The listing builds one solid part. Answer for the finished solid, in the listing's coordinates (mm). A direction names the side the tool comes from. Round coordinates to 2 decimals unless told otherwise and drop trailing zeros. Write each loop counter-clockwise with the first axis right and the second up, starting at its lowest first coordinate (ties: lowest second). Pieces come first, ordered by that corner, then holes.
(1) Find the intervals of material crossed by probe 1 along X at (y, z) = (-11.5, 9.75); probe 2 along Y at (x, z) = (4, 2.25); probe 3 along Y at (x, z) = (15.65, 5), in increasing order.
(2) Each of these flat-tipped pins is pushed along its axis until it touches: pin 1 Ø5 at (y, z) = (-10.5, 5) entering from -X; pin 2 Ø3 at (y, z) = (-47, 7.5) entering from -X; pin 3 Ø0.6 at (y, z) = (-84.5, 0.5) entering from -X. Where does it stop, or does it pass through?
(3) A cutting plane is placed at C-C, the plane z = 5. Give the number of separate pieces and of enclosed holes in the cut face, and give its area (3 significant figures).
(4) A cutting plane is placed at B-B, the plane y = 10. Give the vertices of the cut face in (x, z), and give its area (3 significant figures).
(5) A cutting plane is placed at A-A, the plane y = -10.5. Give the vertices of the cut face in (x, z).
(6) For faces 4 (the face through (15.33, 39.996, 2.708)), 5 (the face through (9, -3, 5)), 6 (the face through (6.844, -85.028, 6.508)), determine the directions among +Z, -Z, +X, -X, +Y, -Y from which every point of the face is accessible in a straight line to the end or side of a thin tool.
(7) The mould has two halves that part along Y. Classify faces 1 (the face through (-0.15, 39.99, 5.07)), 2 (the face through (-0.15, 0.01, 5.07)), 3 (the face through (13.6, -2.4, 10)): +Y half, -Y half, draft (parallel to the pull), parting line (faces both ways), or undercut.
from build123d import *

# Parameters (mm, degrees)
BOSS_EXTRUDE2_DEPTH      = 10
CUT_EXTRUDE2_DEPTH       = 90.877694674
CUT_EXTRUDE2_DEPTH_BACK  = 90.877694674
SKETCH5_W                = 11
SKETCH5_H                = 67.407766248
CUT_EXTRUDE3_DEPTH       = 87.446515257
CUT_EXTRUDE3_DEPTH_BACK  = 87.446515257
SKETCH16_R               = 1.85
FILLET16_R               = 15
CUT_EXTRUDE20_DEPTH      = 92.021975369
CUT_EXTRUDE20_DEPTH_BACK = 92.021975369
SKETCH45_R               = 1.85
SKETCH52_W               = 15
SKETCH52_H               = 10
BOSS_EXTRUDE25_DEPTH     = 4
FILLET17_R               = 10
FILLET18_R               = 2
SKETCH53_R               = 1.9
CUT_EXTRUDE25_DEPTH      = 10
SKETCH55_W               = 0.5
SKETCH55_H               = 4
CUT_EXTRUDE28_DEPTH      = 10
CUT_EXTRUDE32_DEPTH      = 91.055538419
CUT_EXTRUDE32_DEPTH_BACK = 91.055538419
SKETCH60_R               = 2
FILLET19_R               = 10
SKETCH61_R               = 1.85
CUT_EXTRUDE33_DEPTH      = 10


with BuildPart() as part:
    # Sketch2 → Boss-Extrude2 (new body)
    with BuildSketch(Plane.XY):
        Polygon((18, -3), (33, -3), (33, 43), (-3, 43), (-3, -3), (11, -3), (11, -83), (18, -83), align=None)
        Polygon((15, 0), (30, 0), (30, 40), (0, 40), (0, 0), (14, 0), (14, -80), (15, -80), align=None, mode=Mode.SUBTRACT)
    extrude(amount=BOSS_EXTRUDE2_DEPTH)

    # Sketch5 → Cut-Extrude2 (cut, two sides: drawn at the far end of the back side and taken through both)
    with BuildSketch(Plane.XY.offset(10).offset(-CUT_EXTRUDE2_DEPTH_BACK)):
        with Locations((9.5, -51.703883124)):
            Rectangle(SKETCH5_W, SKETCH5_H)
    extrude(amount=CUT_EXTRUDE2_DEPTH + CUT_EXTRUDE2_DEPTH_BACK, mode=Mode.SUBTRACT)

    # Sketch16 → Cut-Extrude3 (cut, two sides: drawn at the far end of the back side and taken through both)
    with BuildSketch(Plane.ZY.offset(-11).offset(-CUT_EXTRUDE3_DEPTH_BACK)):
        with Locations((5, -10.5)):
            Circle(SKETCH16_R)
    extrude(amount=CUT_EXTRUDE3_DEPTH + CUT_EXTRUDE3_DEPTH_BACK, mode=Mode.SUBTRACT)

    # Fillet16
    # the kernel refuses this fillet: 15 mm, written as the material it adds along each edge
    with BuildSketch(Plane(origin=(0, 40, 0), x_dir=(0, -1, 0), z_dir=(0, 0, 1)), Plane(origin=(30, 40, 0), x_dir=(-1, 0, 0), z_dir=(0, 0, 1)), Plane(origin=(30, 0, 0), x_dir=(0, 1, 0), z_dir=(0, 0, 1))) as fillet16_piece_1:
        with BuildLine():
            CenterArc((FILLET16_R, FILLET16_R), FILLET16_R, 180, 90)
            Line((0, FILLET16_R), (-FILLET16_R * 0.02, FILLET16_R))
            Line((-FILLET16_R * 0.02, FILLET16_R), (-FILLET16_R * 0.02, -FILLET16_R * 0.02))
            Line((-FILLET16_R * 0.02, -FILLET16_R * 0.02), (FILLET16_R, -FILLET16_R * 0.02))
            Line((FILLET16_R, -FILLET16_R * 0.02), (FILLET16_R, 0))
        make_face()
    extrude(amount=10)
    with BuildSketch(Plane(origin=(0, 0, 0), x_dir=(1, 0, 0), z_dir=(0, 0, 1))) as fillet16_piece_2:
        with BuildLine():
            CenterArc((15, 14.966629547), FILLET16_R, 180, 86.177446271)
            Line((0, 14.966629547), (-0.3, 14.966629547))
            Line((-0.3, 14.966629547), (-0.3, 0))
            Line((-0.3, 0), (0, -0.3))
            ThreePointArc((0, -0.3), (7, -0.3), (13.98, -0.299332591))
            Line((13.98, -0.299332591), (14, 0))
        make_face()
    extrude(amount=10)

    # Sketch45 → Cut-Extrude20 (cut, two sides: drawn at the far end of the back side and taken through both)
    with BuildSketch(Plane.ZY.offset(3).offset(-CUT_EXTRUDE20_DEPTH_BACK)):
        with Locations((5, 20)):
            Circle(SKETCH45_R)
    extrude(amount=CUT_EXTRUDE20_DEPTH + CUT_EXTRUDE20_DEPTH_BACK, mode=Mode.SUBTRACT)

    # Sketch52 → Boss-Extrude25 (add)
    with BuildSketch(Plane.XZ.offset(83)):
        with Locations((10.5, 5)):
            Rectangle(SKETCH52_W, SKETCH52_H)
    extrude(amount=BOSS_EXTRUDE25_DEPTH)

    # Fillet17
    fillet17_edges = [part.edges().sort_by_distance(p)[0] for p in [
        (-3, -3, 5),
        (33, -3, 5),
    ]]
    fillet(fillet17_edges, radius=FILLET17_R)

    # Fillet18
    fillet18_edges = [part.edges().sort_by_distance(p)[0] for p in [
        (18, -87, 5),
    ]]
    fillet(fillet18_edges, radius=FILLET18_R)

    # Sketch53 → Cut-Extrude25 (cut)
    with BuildSketch(Plane.XZ.offset(87)):
        with Locations(Location((8, 5, 0), (0, 0, 270))):
            Circle(SKETCH53_R)
    extrude(amount=-CUT_EXTRUDE25_DEPTH, mode=Mode.SUBTRACT)

    # Sketch55 → Cut-Extrude28 (cut)
    with BuildSketch(Plane.ZY.offset(-3)):
        with Locations((0.25, -85)):
            Rectangle(SKETCH55_W, SKETCH55_H)
    extrude(amount=-CUT_EXTRUDE28_DEPTH, mode=Mode.SUBTRACT)

    # Sketch60 → Cut-Extrude32 (cut, two sides: drawn at the far end of the back side and taken through both)
    with BuildSketch(Plane(origin=(18, 0, 0), x_dir=(0, 0, -1), z_dir=(1, 0, 0)).offset(-CUT_EXTRUDE32_DEPTH_BACK)):
        with Locations((-5, -10.5)):
            Circle(SKETCH60_R)
    extrude(amount=CUT_EXTRUDE32_DEPTH + CUT_EXTRUDE32_DEPTH_BACK, mode=Mode.SUBTRACT)

    # Fillet19
    fillet19_edges = [part.edges().sort_by_distance(p)[0] for p in [
        (-3, 43, 5),
        (33, 43, 5),
    ]]
    fillet(fillet19_edges, radius=FILLET19_R)

    # Sketch61 → Cut-Extrude33 (cut)
    with BuildSketch(Plane(origin=(0, 43, 0), x_dir=(1, 0, 0), z_dir=(0, 1, 0))):
        with Locations(Location((15, -5, 0), (0, 0, 270))):
            Circle(SKETCH61_R)
    extrude(amount=-CUT_EXTRUDE33_DEPTH, mode=Mode.SUBTRACT)


solid = part.part
Solutions:
1. probe 1: x = 11 to 14, 15 to 18
1. probe 2: y = -87 to -83, -2.54 to 4.77, 35.2 to 42.54
1. probe 3: y = -87 to -12.5, -8.5 to 0.01
2. pin 1: stops at x = 11
2. pin 2: stops at x = 15
2. pin 3: stops at x = 3
3. separate pieces: 7
3. enclosed holes: 0
3. area: 831 mm2
4. outline: (-3, 0) - (0.85, 0) - (0.85, 10) - (-3, 10) - close; (29.14, 0) - (33, 0) - (33, 10) - (29.14, 10) - close
4. area: 77.0 mm2
5. outline: (11, 0) - (14, 0) - (14, 3) - (11, 3) - close; (11, 7) - (14, 7) - (14, 10) - (11, 10) - close; (15, 0) - (18, 0) - (18, 3) - (15, 3) - close; (15, 7) - (18, 7) - (18, 10) - (15, 10) - close
6. face 4: +Z, -Z
6. face 5: +Z, -Z, -X
6. face 6: -Y
7. face 1: +Y half
7. face 2: undercut
7. face 3: draft
